Input: dimensioned drawing with shaded views. Units: mm. Origin: part minimum x, y, z. A direction names the side the tool comes from. Coordinates: 2 decimals unless noted, no trailing zeros. Loops run counter-clockwise (first coordinate to the right, second up) from the corner with the lowest first, then second, coordinate; pieces in that order, holes last.
(1) Section A-A, the plane x = 6.5. Return loops of the section in (y, z).
(2) Line query: L1, parallel to Y at x = 8, z = 1.45; L2, parallel to Y at x = 1, z = 1.45; L3, parallel to X at y = 6, z = 2.15. Output: solid intervals per line, ascending.
(3) Section B-B, the plane y = 5. Return loops of the section in (x, z).
(4) Mould query, pull axis X, two halves, no side actions, for the marked faces 3, 4 and 5. Classes: released by +X, released by -X, zero draft, split by the parting line, or undercut.
(5) Set-up query: the marked faces 1 and 2. Return all of +Z, -Z, +X, -X, +Y, -Y with unobstructed straight access to the full face (end or side cutting, diameter ignored); none if empty.
(6) Section C-C, the plane z = 0.85. Return loops of the section in (x, y).
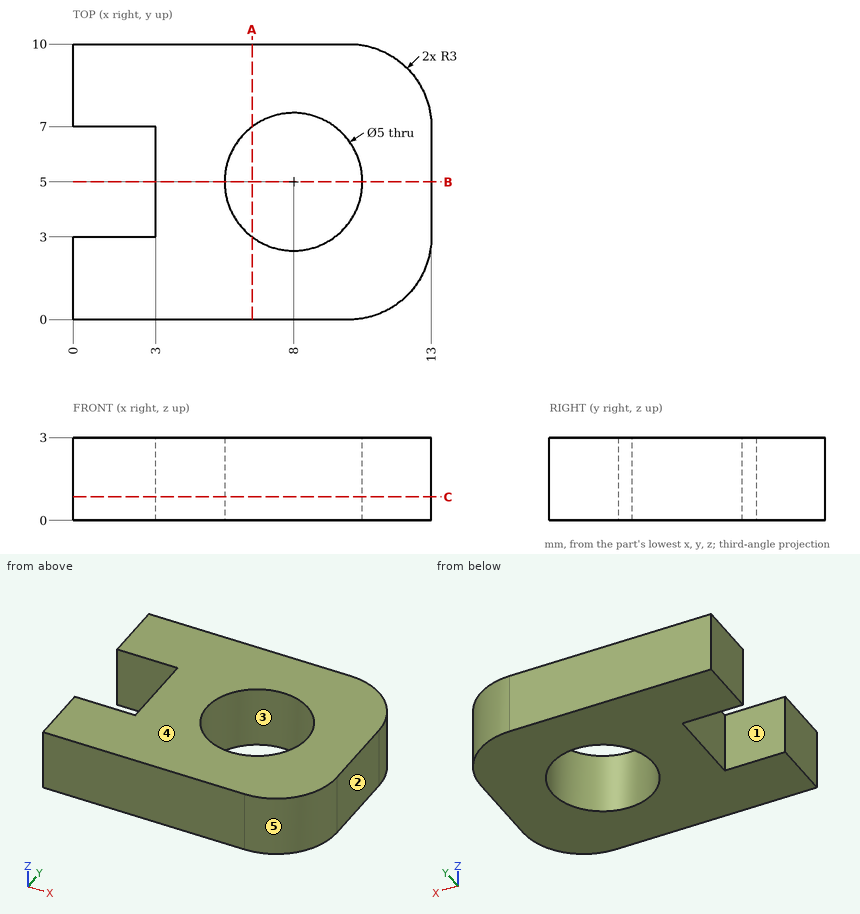
Report:
1. outline: (0, 0) - (3, 0) - (3, 3) - (0, 3) - close; (7, 0) - (10, 0) - (10, 3) - (7, 3) - close
2. L1: y = 0 to 2.5, 7.5 to 10
2. L2: y = 0 to 3, 7 to 10
2. L3: x = 3 to 5.71, 10.29 to 13
3. outline: (3, 0) - (5.5, 0) - (5.5, 3) - (3, 3) - close; (10.5, 0) - (13, 0) - (13, 3) - (10.5, 3) - close
4. face 3: undercut
4. face 4: zero draft
4. face 5: released by +X
5. face 1: +Z, -Z, -X
5. face 2: +Z, -Z, +X, +Y, -Y
6. outline: (0, 0) - (10, 0) arc R3 ccw to (13, 3) - (13, 7) arc R3 ccw to (10, 10) - (0, 10) - (0, 7) - (3, 7) - (3, 3) - (0, 3) - close; hole circle Ø5 at (8, 5)
